```python
from build123d import *

# Parameters (mm, degrees)
BOSS_EXTRUDE1_DEPTH = 20
SKETCH2_W           = 20
SKETCH2_H           = 8
CUT_EXTRUDE1_DEPTH  = 2
SKETCH4_W           = 15
SKETCH4_H           = 35
CUT_EXTRUDE2_DEPTH  = 22
SKETCH5_R           = 1.5
SKETCH5_R_2         = 5.5
CUT_EXTRUDE3_DEPTH  = 20
SKETCH6_R           = 1.5
CUT_EXTRUDE4_DEPTH  = 2
CUT_EXTRUDE5_DEPTH  = 3


with BuildPart() as part:
    # Sketch1 → Boss-Extrude1 (new body)
    with BuildSketch(Plane.XY):
        Polygon((-13, 0), (13, 0), (13, 38), (9, 38), (-13, 3), align=None)
    extrude(amount=BOSS_EXTRUDE1_DEPTH)

    # Sketch2 → Cut-Extrude1 (cut)
    with BuildSketch(Plane(origin=(13, 0, 0), x_dir=(0, 0, -1), z_dir=(1, 0, 0))):
        with Locations((-10, 10)):
            Rectangle(SKETCH2_W, SKETCH2_H)
        with Locations((-10, 26)):
            Rectangle(SKETCH2_W, SKETCH2_H)
    extrude(amount=-CUT_EXTRUDE1_DEPTH, mode=Mode.SUBTRACT)

    # Sketch4 → Cut-Extrude2 (cut)
    with BuildSketch(Plane.ZY.offset(13)):
        with Locations((10, 20.5)):
            Rectangle(SKETCH4_W, SKETCH4_H)
    extrude(amount=-CUT_EXTRUDE2_DEPTH, mode=Mode.SUBTRACT)

    # Sketch5 → Cut-Extrude3 (cut)
    with BuildSketch(Plane.XY.offset(20)):
        with Locations((6, 23.5)):
            Circle(SKETCH5_R)
        with Locations((1, 12)):
            Circle(SKETCH5_R_2)
    extrude(amount=-CUT_EXTRUDE3_DEPTH, mode=Mode.SUBTRACT)

    # Sketch6 → Cut-Extrude4 (cut)
    with BuildSketch(Plane(origin=(11, 0, 0), x_dir=(0, 0, -1), z_dir=(1, 0, 0))):
        with Locations((-10, 26)):
            Circle(SKETCH6_R)
        with Locations((-10, 10)):
            Circle(SKETCH6_R)
    extrude(amount=-CUT_EXTRUDE4_DEPTH, mode=Mode.SUBTRACT)

    # Sketch7 → Cut-Extrude5 (cut)
    with BuildSketch(Plane(origin=(0, 3, 0), x_dir=(1, 0, 0), z_dir=(0, 1, 0))):
        with BuildLine():
            Line((-10, -9), (6, -9))
            ThreePointArc((6, -9), (7, -10), (6, -11))
            Line((6, -11), (-10, -11))
            ThreePointArc((-10, -11), (-11, -10), (-10, -9))
        make_face()
    extrude(amount=-CUT_EXTRUDE5_DEPTH, mode=Mode.SUBTRACT)


solid = part.part
```
Here's how the part is built. I have some questions about the finished solid (model axes, mm). A direction names the side the tool comes from. Coordinates: 2 decimals unless noted, no trailing zeros. Order: outer loops, then holes, each group sorted by start corner. A loop starts at its lowest first (then second) coordinate and runs counter-clockwise, first axis right, second up. Notation, with made-up numbers: (3.25, 48) - (57.25, 48) arc R14 ccw to (57.25, 70) - close; hole circle Ø6 at (-22.5, 20). An arc over 180 degrees is marked (long way). One line per question, with ' | ' between items. Start each with the question number.
1. Which directions (+Z, -Z, +X, -X, +Y, -Y) give clear straight access to the entire face, cutting with the end or side of a thin tool? Please do faces 5 (the flat face through (11, 24, 10)), 6 (the flat face through (0, 0, 8)), 7 (the flat face through (9, 21, 10)).
2. If we mould it in two halves opening along Z, with no side actions, what happens to faces 1 (the flat face through (6, 15, 0)), 2 (the cylindrical face through (-11, 2, 10)), 3 (the flat face through (11, 38, 10)), 4 (the flat face through (-2, 3, 12))? For each: released by +Z, released by -Z, zero draft, split by the parting line, or undercut.
3. I'm going to push flat-ended pins straight in: pin 1 Ø7.5 at (x, z) = (2.5, 10) entering from +Y; pin 2 Ø8 at (x, z) = (4, 11) entering from -Y; pin 3 Ø1.8 at (x, y) = (6, 23.5) entering from -Z; pin 4 Ø5 at (y, z) = (11, 14.5) entering from -X. Where does each tip first touch, or does it pass through?
4. If we section it at D-D (z = 2): Write out the boundary of the cut face in (x, y), and give its area (3 significant figures).
5. Please list where these lines run through material, in increasing order: line 1 along Y through (x, z) = (10.4, 10); line 2 along Z through (x, y) = (-4.25, 9); line 3 along X through (y, z) = (11, 5.5). Write a range as [from, to].
6. If we section it at C-C (x = 1): Write out the boundary of the cut face in (y, z), and give its area (3 significant figures).
7. If we section it at A-A (z = 10): Write out the boundary of the cut face in (x, y), and give its area (3 significant figures).
8. If we section it at B-B (y = 26): Write out the boundary of the cut face in (x, z), and give its area (3 significant figures).
Model answer:
1) face 5: +Z, -Z, +X | face 6: +Z, -Z, +X, -X, -Y | face 7: -X, +Y
2) face 1: released by -Z | face 2: undercut | face 3: zero draft | face 4: undercut
3) pin 1: stops at y = 3 | pin 2: stops at y = 0 | pin 3: passes through | pin 4: stops at x = 9
4) outline: (-13, 0) - (13, 0) - (13, 6) - (11, 6) - (11, 14) - (13, 14) - (13, 22) - (11, 22) - (11, 30) - (13, 30) - (13, 38) - (9, 38) - (-13, 3) - close; hole circle Ø11 at (1, 12); hole circle Ø3 at (6, 23.5) | area: 469 mm²
5) line 1: y = [0, 8.5], [11.5, 24.5], [27.5, 38] | line 2: z = [0, 2.5], [17.5, 20] | line 3: x = [9, 11]
6) outline: (0, 0) - (6.5, 0) - (6.5, 2.5) - (3, 2.5) - (3, 9) - (0, 9) - close; (0, 11) - (3, 11) - (3, 17.5) - (6.5, 17.5) - (6.5, 20) - (0, 20) - close; (17.5, 0) - (25.27, 0) - (25.27, 2.5) - (17.5, 2.5) - close; (17.5, 17.5) - (25.27, 17.5) - (25.27, 20) - (17.5, 20) - close | area: 110 mm²
7) outline: (-13, 0) - (-11, 0) - (-11, 3) - (-13, 3) - close; (7, 0) - (13, 0) - (13, 6) - (11, 6) - (11, 8.5) - (9, 8.5) - (9, 3) - (7, 3) - close; (9, 11.5) - (11, 11.5) - (11, 14) - (13, 14) - (13, 22) - (11, 22) - (11, 24.5) - (9, 24.5) - close; (9, 27.5) - (11, 27.5) - (11, 30) - (13, 30) - (13, 38) - (9, 38) - close | area: 120 mm²
8) outline: (1.46, 0) - (11, 0) - (11, 8.5) - (9, 8.5) - (9, 2.5) - (1.46, 2.5) - close; (1.46, 17.5) - (9, 17.5) - (9, 11.5) - (11, 11.5) - (11, 20) - (1.46, 20) - close | area: 71.7 mm²
